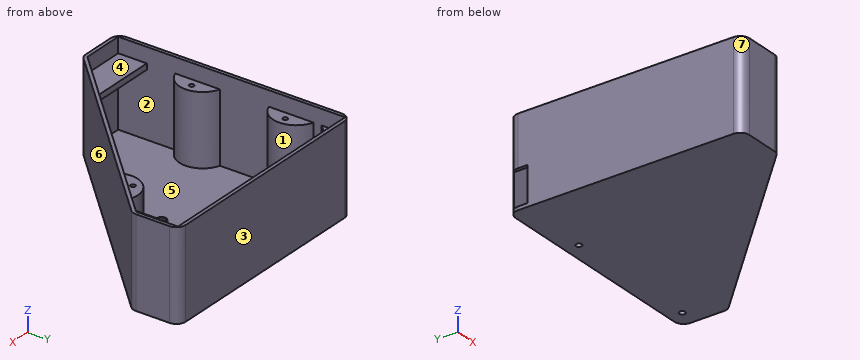
```python
from build123d import *

# Parameters (mm, degrees)
ESTRUSIONE_ESTRUSIONE1_DEPTH  = 80
SVUOTA1_T                     = -3
TAGLIO_ESTRUSIONE1_DEPTH      = 294.938769134
TAGLIO_ESTRUSIONE1_DEPTH_BACK = 294.938769134
SCHIZZO5_W                    = 4
SCHIZZO5_H                    = 200
ESTRUSIONE_ESTRUSIONE4_DEPTH  = 60
SCHIZZO8_R                    = 2
TAGLIO_ESTRUSIONE2_DEPTH      = 30
ESTRUSIONE_ESTRUSIONE7_DEPTH  = 5
ESTRUSIONE_ESTRUSIONE8_DEPTH  = 9
ESTRUSIONE_ESTRUSIONE9_START  = 2
ESTRUSIONE_ESTRUSIONE9_DEPTH  = 2
TAGLIO_ESTRUSIONE3_START      = -3
TAGLIO_ESTRUSIONE3_OUTLINE_W  = 30
TAGLIO_ESTRUSIONE3_OUTLINE_H  = 13
TAGLIO_ESTRUSIONE3_DEPTH      = 3
TAGLIO_ESTRUSIONE5_DEPTH      = 10
SCHIZZO18_R                   = 6
ESTRUSIONE_ESTRUSIONE11_DEPTH = 3
TAGLIO_ESTRUSIONE6_DEPTH      = 292.376045687
TAGLIO_ESTRUSIONE6_DEPTH_BACK = 292.376045687
SCHIZZO19_R                   = 2.5
RACCORDO1_R                   = 8


# Read off the part's stored shape, not the designer's step: Taglio-Estrusione3
with BuildPart() as part:
    # Schizzo2 → Estrusione-Estrusione1 (new body)
    with BuildSketch(Plane.XY):
        Polygon((0, 0), (0, 200), (200, 200), (200, 160), (40, 0), align=None)
    extrude(amount=ESTRUSIONE_ESTRUSIONE1_DEPTH)

    # Svuota1
    svuota1_openings = [part.faces().sort_by_distance(p)[0] for p in [
        (78.039215686, 121.960784314, 80),
    ]]
    offset(amount=SVUOTA1_T, openings=svuota1_openings, kind=Kind.INTERSECTION)

    # Schizzo5 → Taglio-Estrusione1 (cut, two sides: drawn at the far end of the back side and taken through both)
    with BuildSketch(Plane(origin=(200, 0, 0), x_dir=(0, 0, -1), z_dir=(1, 0, 0)).offset(-TAGLIO_ESTRUSIONE1_DEPTH_BACK)):
        with Locations((-78, 100)):
            Rectangle(SCHIZZO5_W, SCHIZZO5_H)
    extrude(amount=TAGLIO_ESTRUSIONE1_DEPTH + TAGLIO_ESTRUSIONE1_DEPTH_BACK, mode=Mode.SUBTRACT)

    # Schizzo7 → Estrusione-Estrusione4 (add)
    with BuildSketch(Plane.XY.offset(63)):
        with BuildLine():
            Line((140.775884186, 105.018524874), (167.757359313, 132))
            ThreePointArc((167.757359313, 132), (144.367126813, 128.408757373), (140.775884186, 105.018524874))
        make_face()
        with BuildLine():
            ThreePointArc((3, 170), (17, 150.921215972), (3, 131.842431943))
            Line((3, 131.842431943), (3, 170))
        make_face()
        with BuildLine():
            ThreePointArc((3, 90), (17, 70.921215972), (3, 51.842431943))
            Line((3, 51.842431943), (3, 90))
        make_face()
    extrude(amount=-ESTRUSIONE_ESTRUSIONE4_DEPTH)

    # Schizzo8 → Taglio-Estrusione2 (cut)
    with BuildSketch(Plane.XY.offset(63)):
        with Locations((10, 150.921215972)):
            Circle(SCHIZZO8_R)
        with Locations((10, 70.921215972)):
            Circle(SCHIZZO8_R)
        with Locations((149.316874281, 123.459009905)):
            Circle(SCHIZZO8_R)
    extrude(amount=-TAGLIO_ESTRUSIONE2_DEPTH, mode=Mode.SUBTRACT)

    # Schizzo11 → Estrusione-Estrusione7 (add)
    with BuildSketch(Plane.XY.offset(63)):
        Polygon((3, 197), (3, 177), (23, 197), align=None)
        Polygon((197, 161.242640687), (197, 197), (177, 197), (177, 141.242640687), align=None)
        Polygon((3, 3), (3, 27.421215972), (63.178575285, 27.421215972), (38.757359313, 3), align=None)
    extrude(amount=-ESTRUSIONE_ESTRUSIONE7_DEPTH)

    # Schizzo12 → Estrusione-Estrusione8 (add)
    with BuildSketch(Plane.XY.offset(72)):
        with BuildLine():
            Line((193, 184), (197, 184))
            Line((197, 184), (197, 176))
            Line((197, 176), (193, 176))
            ThreePointArc((193, 176), (189, 180), (193, 184))
        make_face()
    extrude(amount=-ESTRUSIONE_ESTRUSIONE8_DEPTH)

    # Schizzo13 → Estrusione-Estrusione9 (add)
    with BuildSketch(Plane.XY.offset(72).offset(ESTRUSIONE_ESTRUSIONE9_START)):
        with BuildLine():
            Line((193, 177), (196, 177))
            Line((196, 177), (197, 177))
            Line((197, 177), (197, 176))
            Line((197, 176), (193, 176))
            ThreePointArc((193, 176), (189, 180), (193, 184))
            Line((193, 184), (197, 184))
            Line((197, 184), (197, 183))
            Line((197, 183), (193, 183))
            ThreePointArc((193, 183), (190, 180), (193, 177))
        make_face()
    extrude(amount=-ESTRUSIONE_ESTRUSIONE9_DEPTH)

    # Taglio-Estrusione3 outline → Taglio-Estrusione3 (cut)
    with BuildSketch(Plane(origin=(3, 0, 0), x_dir=(0, 0, -1), z_dir=(1, 0, 0)).offset(TAGLIO_ESTRUSIONE3_START)):
        with Locations((-18, 190.5)):
            Rectangle(TAGLIO_ESTRUSIONE3_OUTLINE_W, TAGLIO_ESTRUSIONE3_OUTLINE_H)
    extrude(amount=TAGLIO_ESTRUSIONE3_DEPTH, mode=Mode.SUBTRACT)

    # Schizzo16 → Taglio-Estrusione5 (cut)
    with BuildSketch(Plane.XY.offset(63)):
        with BuildLine():
            Line((190.171572875, 182.828427125), (177, 169.656854249))
            Line((177, 169.656854249), (177, 197))
            Line((177, 197), (197, 197))
            Line((197, 197), (197, 184))
            Line((197, 184), (193, 184))
            ThreePointArc((193, 184), (191.469266271, 183.69551813), (190.171572875, 182.828427125))
        make_face()
    extrude(amount=-TAGLIO_ESTRUSIONE5_DEPTH, mode=Mode.SUBTRACT)

    # Schizzo18 → Estrusione-Estrusione11 (add)
    with BuildSketch(Plane.XY.offset(3)):
        with Locations(Location((65, 188, 0), (0, 0, 180))):
            Circle(SCHIZZO18_R)
        with Locations(Location((185, 188, 0), (0, 0, 180))):
            Circle(SCHIZZO18_R)
    extrude(amount=ESTRUSIONE_ESTRUSIONE11_DEPTH)

    # Schizzo19 → Taglio-Estrusione6 (cut, two sides: drawn at the far end of the back side and taken through both)
    with BuildSketch(Plane.XY.offset(6).offset(-TAGLIO_ESTRUSIONE6_DEPTH_BACK)):
        with Locations((65, 188)):
            Circle(SCHIZZO19_R)
        with Locations((185, 188)):
            Circle(SCHIZZO19_R)
    extrude(amount=TAGLIO_ESTRUSIONE6_DEPTH + TAGLIO_ESTRUSIONE6_DEPTH_BACK, mode=Mode.SUBTRACT)

    # Raccordo1
    # the kernel refuses this fillet: 8 mm, written as the material it takes off along each edge
    with BuildSketch(Plane(origin=(40, 0, -8.284271247), x_dir=(-1, 0, 0), z_dir=(0, 0, 1)), Plane(origin=(200, 160, -8.284271247), x_dir=(-0.7071067811865432, -0.7071067811865518, 0), z_dir=(0, 0, 1))) as raccordo1_piece_1:
        with BuildLine():
            CenterArc((RACCORDO1_R * 0.414213562373, -RACCORDO1_R), RACCORDO1_R, 90, 45)
            Line((-RACCORDO1_R * 0.292893218813, -RACCORDO1_R * 0.292893218813), (0, 0))
            Line((0, 0), (RACCORDO1_R * 0.414213562373, 0))
        make_face()
    extrude(amount=92.568542495, mode=Mode.SUBTRACT)
    with BuildSketch(Plane(origin=(0, 0, -20), x_dir=(0, 1, 0), z_dir=(0, 0, 1))) as raccordo1_piece_2:
        with BuildLine():
            CenterArc((RACCORDO1_R, -RACCORDO1_R), RACCORDO1_R, 90, 90)
            Line((0, -RACCORDO1_R), (0, 0))
            Line((0, 0), (RACCORDO1_R, 0))
        make_face()
    extrude(amount=116, mode=Mode.SUBTRACT)
    with BuildSketch(Plane(origin=(0, 200, -20), x_dir=(0, -1, 0), z_dir=(0, 0, 1)), Plane(origin=(200, 200, -20), x_dir=(-1, 0, 0), z_dir=(0, 0, 1))) as raccordo1_piece_3:
        with BuildLine():
            CenterArc((RACCORDO1_R, RACCORDO1_R), RACCORDO1_R, 180, 90)
            Line((0, RACCORDO1_R), (0, 0))
            Line((0, 0), (RACCORDO1_R, 0))
        make_face()
    extrude(amount=116, mode=Mode.SUBTRACT)


solid = part.part
```
Input: part model. Units: mm. Frame: model coordinates. Face numbers are marked on the shaded views. A direction names the side the tool comes from. Round coordinates to 2 decimals unless told otherwise and drop trailing zeros. Order: outer loops, then holes, each group sorted by start corner. A loop starts at its lowest first (then second) coordinate and runs counter-clockwise, first axis right, second up. Notation, with made-up numbers: (3, -39) - (41, -39) arc R28 cw to (41, -5) - close; hole circle Ø1 at (-33.5, -39). An arc over 180 degrees is marked (long way). One line per question, with ' | ' between items. Start each with the question number.
1) Cut plane C-C, the plane z = 50. Return the cut outline in (x, y), then the cut area to 3 significant figures.
2) Cut plane B-B, the plane z = 69. Return the cut outline in (x, y).
3) Pull-direction query (X, two-part tool) for the marked faces 4, 5, 6 and 7; classes: +X half, -X half, draft (parallel to the pull), parting line (faces both ways), or undercut.
4) Ray query, probe 1 along X at (y, z) = (188, 4.85); probe 2 along X at (y, z) = (179, 39.5); probe 3 along Y at (x, z) = (185, 3.55). Return the intervals inside material, ascending.
5) Cut plane A-A, the plane y = 188. Give the number of separate pieces and of enclosed holes in the cut face, then the cut area to 4 significant figures.
6) Cut plane D-D, the plane x = 118. Return the cut outline in (y, z), then the cut area to 3 significant figures.
7) Set-up query: the marked faces 1, 2 and 3. Return all of +Z, -Z, +X, -X, +Y, -Y with unobstructed straight access to the full face (end or side cutting, diameter ignored); none if empty.
8) Contact query for flat-ended pins moving along their axis: P1, Ø1.6, axis at x = 195, z = 73, coming from the +Y side; P2, Ø4, axis at y = 128.5, z = 31.5, coming from the +X side; P3, Ø2, axis at x = 59.5, z = 47, coming from the -Y side. Output: stop coordinate, or through.
Worked out:
1) outline: (0, 8) arc R8 ccw to (8, 0) - (36.69, 0) arc R8 ccw to (42.34, 2.34) - (197.66, 157.66) arc R8 ccw to (200, 163.31) - (200, 192) arc R8 ccw to (192, 200) - (8, 200) arc R8 ccw to (0, 192) - close; hole (3, 3) - (38.76, 3) - (140.78, 105.02) arc R20 cw to (167.76, 132) - (197, 161.24) - (197, 197) - (3, 197) - (3, 170) arc R20 cw to (3, 131.84) - (3, 90) arc R20 cw to (3, 51.84) - close; hole circle Ø4 at (10, 70.92); hole circle Ø4 at (10, 150.92); hole circle Ø4 at (149.32, 123.46) | area: 3,180 mm^2
2) outline: (0, 8) arc R8 ccw to (8, 0) - (36.69, 0) arc R8 ccw to (42.34, 2.34) - (197.66, 157.66) arc R8 ccw to (200, 163.31) - (200, 192) arc R8 ccw to (192, 200) - (8, 200) arc R8 ccw to (0, 192) - close; hole (3, 3) - (38.76, 3) - (197, 161.24) - (197, 176) - (193, 176) arc R4 cw to (193, 184) - (197, 184) - (197, 197) - (3, 197) - close
3) face 4: undercut | face 5: undercut | face 6: +X half | face 7: -X half
4) probe 1: x = 59 to 62.5, 67.5 to 71, 179 to 182.5, 187.5 to 191, 197 to 200 | probe 2: x = 0 to 3, 197 to 200 | probe 3: y = 145 to 149.24, 182 to 185.5, 190.5 to 194, 197 to 200
5) separate pieces: 4 | enclosed holes: 0 | area: 1,015 mm^2
6) outline: (78, 0) - (200, 0) - (200, 76) - (197, 76) - (197, 3) - (82.24, 3) - (82.24, 76) - (78, 76) - close | area: 895 mm^2
7) face 1: +Z | face 2: none | face 3: +Z, -Z, +X, -X, +Y
8) P1: stops at y = 199.69 | P2: stops at x = 170.5 | P3: stops at y = 18.5
